The listing builds one solid part. Answer for the finished solid, in the listing's coordinates (mm). Coordinates: 2 decimals unless noted, no trailing zeros. Write each loop counter-clockwise with the first axis right and the second up, starting at its lowest first coordinate (ties: lowest second). Pieces come first, ordered by that corner, then holes.
from build123d import *

# Parameters (mm, degrees)
F1_DEPTH = 6.8
F2_R     = 4
F3_DEPTH = 6.801


with BuildPart() as f1:
    # F0 (on Front) → F1 (new body)
    with BuildSketch(Plane.XZ):
        Polygon((3.752777, -6.5), (7.505553, 0), (3.752777, 6.5), (-3.752777, 6.5), (-7.505553, 0), (-3.752777, -6.5), align=None)
    extrude(amount=F1_DEPTH)

    # F2 (on face) → F3 (cut, through all)
    with BuildSketch(Plane.XZ.offset(6.8)):
        Circle(F2_R)
    extrude(amount=-F3_DEPTH, mode=Mode.SUBTRACT)


solid = f1.part
Q1. The part is cut by section A-A, the plane z = -3.25. Write down the section's boundary in (x, y), then the cut area to 3 significant figures.
Answers below:
outline: (-5.63, -6.8) - (-2.33, -6.8) - (-2.33, 0) - (-5.63, 0) - close; (2.33, -6.8) - (5.63, -6.8) - (5.63, 0) - (2.33, 0) - close
area: 44.8 mm2
Q2. Given pin 1 (1 mm diameter, centred on x = -1.5, z = 2.5, fed in from -Y); pin 2 (2 mm diameter, centred on y = -1, z = 3, fed in from +X), each flat-ended and moving along its own axis, determine where each tip first touches the part or whether it passes through.
Answers below:
pin 1: passes through
pin 2: stops at x = 6.35
Q3. Determine the mould class of faces 1 (the face through (5.6, -3.4, -3.3)), 2 (the face through (3, 0, -3)), 3 (the face through (3, -6.8, -3)) for opening direction Y: released by +Y, released by -Y, zero draft, split by the parting line, or undercut.
Answers below:
face 1: zero draft
face 2: released by +Y
face 3: released by -Y
Q4. The part is cut by section B-B, the plane x = 0. Write down the section's boundary in (y, z), then the cut area to 3 significant figures.
Answers below:
outline: (-6.8, -6.5) - (0, -6.5) - (0, -4) - (-6.8, -4) - close; (-6.8, 4) - (0, 4) - (0, 6.5) - (-6.8, 6.5) - close
area: 34.0 mm2
Q5. Find the intervals of material crossed by probe 1 along Z at (x, y) = (0, -4.5); probe 2 along X at (y, z) = (-4, 1.5); probe 3 along X at (y, z) = (-3, -1), in increasing order.
Answers below:
probe 1: z = -6.5 to -4, 4 to 6.5
probe 2: x = -6.64 to -3.71, 3.71 to 6.64
probe 3: x = -6.93 to -3.87, 3.87 to 6.93
Q6. The part is cut by section D-D, the plane x = -6. Write down the section's boundary in (y, z), then the cut area to 3 significant figures.
Answers below:
outline: (-6.8, -2.61) - (0, -2.61) - (0, 2.61) - (-6.8, 2.61) - close
area: 35.5 mm2
Q7. The part is cut by section C-C, the plane y = -4.5. Write down the section's boundary in (x, z).
Answers below:
outline: (-7.51, 0) - (-3.75, -6.5) - (3.75, -6.5) - (7.51, 0) - (3.75, 6.5) - (-3.75, 6.5) - close; hole circle Ø8 at (0, 0)
